Autodesk Inventor part; units mm, degrees
ref_plane "YZ Plane" through (0, 0, 0) normal (1, 0, 0) x (0, 1, 0)
ref_plane "XZ Plane" through (0, 0, 0) normal (0, 1, 0) x (-1, 0, 0)
ref_plane "XY Plane" through (0, 0, 0) normal (0, 0, 1) x (1, 0, 0)
sketch "Sketch1" plane through (0, 0, 0) normal (0, 1, 0) x (-1, 0, 0)
  line L0 (0, 0) -> (-25.4, 0)
  line L1 (-25.4, 0) -> (-25.4, -25.4)
  line L2 (-25.4, -25.4) -> (0, -25.4)
  line L3 (0, -25.4) -> (0, 0)
  dimension "d0" = 25.4
extrude "Extrusion1" add sketch "Sketch1" along normal blind 6.35
sketch "Sketch2" plane through (0, 6.35, 0) normal (0, 1, 0) x (1, 0, 0)
  circle A0 centre (8.4667, 13.97) radius 0.635
  circle A1 centre (16.9333, 13.97) radius 0.635
  circle A2 centre (16.9333, 11.43) radius 0.635
  circle A3 centre (8.4667, 11.43) radius 0.635
  line L0 (25.4, 0) -> (25.4, 25.4)
  line L1 (0, 0) -> (25.4, 0)
  dimension "d3" = 8.4667
  dimension "d4" = 8.4667
  dimension "d5" = 2.54
  dimension "d6" = 1.27
  dimension "d7" = 11.43
extrude "Extrusion2" cut sketch "Sketch2" against normal blind 6.35
sketch "Sketch4" plane through (0, 0, 0) normal (0, -1, 0) x (1, 0, 0)
  line L0 (25.4, -25.4) -> (0, -25.4)
  arc A0 (9.525, -25.4) -> (15.875, -25.4) centre (12.7, -28.575) ccw
  line L1 (15.875, -25.4) -> (9.525, -25.4)
  point P0 (0, 0)
  dimension "d10" = 90
  dimension "d11" = 6.35
  dimension "d12" = 9.525
extrude "Extrusion3" add sketch "Sketch4" against normal blind 3.175
sketch "Sketch6" plane through (0, 0, 0) normal (0, -1, 0) x (1, 0, 0)
  line L0 (25.4, 0) -> (25.4, -25.4)
  arc A0 (25.4, -9.525) -> (25.4, -15.875) centre (22.225, -12.7) ccw
  line L1 (25.4, -15.875) -> (25.4, -9.525)
  point P0 (0, 0)
  dimension "d21" = 6.35
  dimension "d22" = 90
  dimension "d23" = 9.525
extrude "Extrusion5" cut sketch "Sketch6" against normal blind 3.175
sketch "Sketch7" plane through (0, 0, 0) normal (0, -1, 0) x (1, 0, 0)
  line L0 (0, -25.4) -> (0, 0)
  arc A0 (0, -9.525) -> (0, -15.875) centre (-3.175, -12.7) ccw
  line L1 (0, -15.875) -> (0, -9.525)
  dimension "d26" = 6.35
  dimension "d27" = 90
  dimension "d28" = 9.525
extrude "Extrusion6" add sketch "Sketch7" against normal blind 3.175
sketch "Sketch8" plane through (0, 0, 0) normal (0, -1, 0) x (1, 0, 0)
  line L0 (0, 0) -> (25.4, 0)
  arc A0 (9.525, 0) -> (15.875, 0) centre (12.7, -3.175) ccw
  line L1 (15.875, 0) -> (9.525, 0)
  dimension "d31" = 90
  dimension "d32" = 6.35
  dimension "d33" = 9.525
extrude "Extrusion7" cut sketch "Sketch8" against normal blind 3.175
equation "\"d1\" = 0.25 * d0"
equation "\"d3\" = 0.333333 * d0"
equation "\"d4\" = d3"
equation "\"d8\" = 0.25 * d0"
equation "\"d11\" = 0.25 * d0"
equation "\"d12\" = 0.375 * d0"
equation "\"d13\" = 0.5 * d1"
equation "\"d21\" = 0.25 * d0"
equation "\"d23\" = 0.375 * d0"
equation "\"d24\" = 0.5 * d1"
equation "\"d26\" = 0.25 * d0"
equation "\"d28\" = 0.375 * d0"
equation "\"d29\" = 0.5 * d1"
equation "\"d32\" = 0.25 * d0"
equation "\"d33\" = 0.375 * d0"
equation "\"d34\" = 0.5 * d1"
properties part number "pieceBase"
Check sheet for the modelled part. Datum: model origin and axes. Units: mm. A direction names the side the tool comes from. Coordinates: 2 decimals unless noted, no trailing zeros. Write each loop counter-clockwise with the first axis right and the second up, starting at its lowest first coordinate (ties: lowest second). Pieces come first, ordered by that corner, then holes. Notation, with made-up numbers: M -38,-36.75 L -7,-36.75 A22 cw -7,-12.75 Z; hole C -37,1.5 d5. An arc over 180 degrees is marked long. Write item = value, one per line. Start each with the question number.
1. Sectioned sample at A-A (x = 12.7). Record the cut outline in (y, z) (3 decimals), then the cut area to 3 significant figures.
2. Sectioned sample at C-C (y = 1). Record the cut outline in (x, z) (3 decimals), then the cut area to 3 significant figures.
3. Tool access check on faces 5 (the flat face through (-4, 3.175, -13)), 6 (the flat face through (9, 0, -16)), 7 (the flat face through (22, 3.175, -13)). Record the directions out of +Z, -Z, +X, -X, +Y, -Y that give a thin tool (end or side, any length) a straight path to the whole face; none if there is none.
4. Sectioned sample at D-D (z = -3). Record the cut outline in (x, y) (3 decimals), then the cut area to 3 significant figures.
5. Go/stop test with flat-tipped pins: pin 1 (1.9 mm diameter, centred on y = 2, z = -16, fed in from -X); pin 2 (2.5 mm diameter, centred on x = 11.5, z = -28.5, fed in from +Y) (3 decimals); pin 3 (1.1 mm diameter, centred on x = 16.93, z = -13.97, fed in from -Y); pin 4 (1.5 mm diameter, centred on x = 21, z = -10, fed in from -Y) (3 decimals). Record where each tip stops, or that it passes through.
6. Mould release check, pull along X, two halves, no side actions. Record for faces 1 (the cylindrical face through (16.3, 3.2, -14)), 2 (the cylindrical face through (16.465, 3.219, -11.859)), 3 (the flat face through (13, 3.175, -29)), 4 (the flat face through (25.4, 4, -13)): pulls with the +X half, pulls with the -X half, needs draft (parallel to the pull), parting line crosses it, or undercut.
7. Sectioned sample at B-B (z = -11.43). Record the cut outline in (x, y) (3 decimals).
8. Thickness scan on probe 1 along X at (y, z) = (5.25, -13.97); probe 2 along X at (y, z) = (0.75, -14); probe 3 along Y at (x, z) = (20, -13.5) (3 decimals). Record the ranges inside material, lowest first.
The answers:
q1.outline = M 0,-33.065 L 3.175,-33.065 L 3.175,-25.4 L 6.35,-25.4 L 6.35,0 L 3.175,0 L 3.175,-7.665 L 0,-7.665 Z
q1.area = 161 mm²
q2.outline = M 0,-25.4 L 9.525,-25.4 A4.49 ccw long 15.875,-25.4 L 25.4,-25.4 L 25.4,-15.875 A4.49 cw long 25.4,-9.525 L 25.4,0 L 15.875,0 A4.49 cw long 9.525,0 L 0,0 L 0,-9.525 A4.49 ccw long 0,-15.875 Z; hole C 8.467,-13.97 d1.27; hole C 8.467,-11.43 d1.27; hole C 16.933,-13.97 d1.27; hole C 16.933,-11.43 d1.27
q2.area = 640 mm²
q3.face_5 = +Z, -Z, -X, +Y
q3.face_6 = +Z, -Z, +X, -X, -Y
q3.face_7 = -Y
q4.outline = M 0,0 L 8.213,0 L 8.213,3.175 L 17.187,3.175 L 17.187,0 L 25.4,0 L 25.4,6.35 L 0,6.35 Z
q4.area = 133 mm²
q5.pin_1 = -7
q5.pin_2 = 3.175
q5.pin_3 = through
q5.pin_4 = 3.175
q6.face_1 = undercut
q6.face_2 = undercut
q6.face_3 = needs draft
q6.face_4 = pulls with the +X half
q7.outline = M -7.482,0 L 7.832,0 L 7.832,6.35 L 0,6.35 L 0,3.175 L -7.482,3.175 Z; M 9.102,0 L 16.298,0 L 16.298,6.35 L 9.102,6.35 Z; M 17.568,0 L 17.918,0 L 17.918,3.175 L 25.4,3.175 L 25.4,6.35 L 17.568,6.35 Z
q8.probe_1 = 0 to 7.83, 9.1 to 16.3, 17.57 to 25.4
q8.probe_2 = -7.47 to 7.83, 9.1 to 16.3, 17.57 to 17.93
q8.probe_3 = 3.175 to 6.35
